Input: part model. Units: mm. Frame: model coordinates. A direction names the side the tool comes from. Round coordinates to 2 decimals unless told otherwise and drop trailing zeros. Loops run counter-clockwise (first coordinate to the right, second up) from the corner with the lowest first, then second, coordinate; pieces in that order, holes last. Notation, with made-up numbers: M -20,39 L -7,39 A29 ccw -7,72 Z; hole C -24,71.5 d5. An arc over 180 degrees is marked long. Return JSON: item names as keys, results as strings. Group by question number.
1) Contact query for flat-ended pins moving along their axis: P1, Ø2, axis at y = 7.5, z = -35.5, coming from the +X side; P2, Ø7.5, axis at x = -43, z = -15.5, coming from the +Y side; P3, Ø5, axis at x = -40.5, y = 32, coming from the -Z side; P4, Ø5, axis at x = 7.5, y = 15, coming from the +Z side. Output: stop coordinate, or through.
2) Access query for faces 5 (the face through (0, 0, -42)), 6 (the face through (0, 2, -44)), 7 (the face through (36.6, 35, -17)), 8 (the face through (-42, 36, -1.65)). Directions: +Z, -Z, +X, -X, +Y, -Y. A direction counts if a zero-diameter tool reaches every point of the face in a straight line with its end or side. Return the directions, or none.
3) Material intervals for line 1 (X direction, y = 28, z = -4); line 2 (Y direction, x = -21, z = -35.5); line 3 (X direction, y = 32.5, z = -5.5), sorted ascending. Write a range as from..to.
4) Section C-C (y = 7). Output: boundary loops of the cut face in (x, z), plus the area to 3 significant figures.
5) Mould query, pull axis Y, two halves, no side actions, for faces 1 (the face through (41, 53, 0)), 2 (the face through (-40, 49, -14)), 3 (the face through (42, 2, -14)), 4 (the face through (-41, 36, -5.65)). Classes: +Y half, -Y half, draft (parallel to the pull), parting line (faces both ways), or undercut.
6) Section B-B (y = 23.5). Output: boundary loops of the cut face in (x, z).
7) Section A-A (y = 42.5). Output: boundary loops of the cut face in (x, z).
from build123d import *

# Parameters (mm, degrees)
EXTRUDE_1_DEPTH          = 58
FILLET_1_R               = 5
SKETCH_2_W               = 14.1984483
SKETCH_2_H               = 27
CUT_EXTRUDE_1_DEPTH      = 1.65
CUT_EXTRUDE_START        = -22.111141
SKETCH_3_R               = 1.5
CUT_EXTRUDE_2_DEPTH      = 22.111141
SKETCH_5_W               = 9.9
SKETCH_5_H               = 27
CUT_EXTRUDE_3_DEPTH      = 22.65
FILLET_2_R               = 1
EXTRUDE_2_DEPTH          = 10
SKETCH_9_R               = 1
CUT_EXTRUDE_4_DEPTH      = 2
PATTERN_CIRCULAR_1_COUNT = 5


with BuildPart() as part:
    # 草图1 → 凸台-拉伸1 (new body)
    with BuildSketch(Plane(origin=(0, 0, 0), x_dir=(1, 0, 0), z_dir=(0, 1, 0))):
        with BuildLine():
            Line((-46.5, 0), (-36.6, 0))
            ThreePointArc((-36.6, 0), (0, 36.6), (36.6, 0))
            Line((36.6, 0), (46.5, 0))
            ThreePointArc((46.5, 0), (0, 46.5), (-46.5, 0))
        make_face()
    extrude(amount=EXTRUDE_1_DEPTH)

    # 圆角1
    fillet_1_edges = [part.edges().sort_by_distance(p)[0] for p in [
        (0, 0, -36.6),
    ]]
    fillet(fillet_1_edges, radius=FILLET_1_R)

    # 草图2 → 切除-拉伸1 (cut)
    with BuildSketch(Plane.XY):
        with Locations((-41.149885232, 35.5)):
            Rectangle(SKETCH_2_W, SKETCH_2_H)
    cut_extrude_1 = extrude(amount=-CUT_EXTRUDE_1_DEPTH, mode=Mode.SUBTRACT)

    # 草图3 → 切除-拉伸2 (cut)
    with BuildSketch(Plane.XY.offset(-1.65).offset(CUT_EXTRUDE_START)):
        with Locations((-41.470716586, 28.5)):
            Circle(SKETCH_3_R)
        with Locations((-41.470716586, 42.5)):
            Circle(SKETCH_3_R)
    cut_extrude_2 = extrude(amount=CUT_EXTRUDE_2_DEPTH, mode=Mode.SUBTRACT)

    # 草图5 → 切除-拉伸3 (cut)
    with BuildSketch(Plane.XY.offset(-5.65)):
        with Locations((-41.55, 35.5)):
            Rectangle(SKETCH_5_W, SKETCH_5_H)
    cut_extrude_3 = extrude(amount=-CUT_EXTRUDE_3_DEPTH, mode=Mode.SUBTRACT)

    # 镜向2: 切除-拉伸1, 切除-拉伸2, 切除-拉伸3 across plane
    add(cut_extrude_1.mirror(Plane(origin=(0, 0, 0), x_dir=(0, 0, 1), z_dir=(1, 0, 0))), mode=Mode.SUBTRACT)
    add(cut_extrude_2.mirror(Plane(origin=(0, 0, 0), x_dir=(0, 0, 1), z_dir=(1, 0, 0))), mode=Mode.SUBTRACT)
    add(cut_extrude_3.mirror(Plane(origin=(0, 0, 0), x_dir=(0, 0, 1), z_dir=(1, 0, 0))), mode=Mode.SUBTRACT)

    # 圆角2
    fillet_2_edges = [part.edges().sort_by_distance(p)[0] for p in [
        (0, 58, -46.5),
    ]]
    fillet(fillet_2_edges, radius=FILLET_2_R)

    # 草图8 → 凸台-拉伸2 (add)
    with BuildSketch(Plane.XZ):
        with BuildLine():
            Line((0, -41.6), (0, -46.5))
            ThreePointArc((0, -46.5), (-2.433621965, -46.436273366), (-4.860573542, -46.245268135))
            Line((-4.860573542, -46.245268135), (-4.348384072, -41.372110847))
            ThreePointArc((-4.348384072, -41.372110847), (-2.17717578, -41.542988646), (0, -41.6))
        make_face()
    extrude(amount=-EXTRUDE_2_DEPTH)

    # 草图9 → 切除-拉伸4 (cut)
    with BuildSketch(Plane.XZ):
        with Locations((0, -44.5)):
            Circle(SKETCH_9_R)
    cut_extrude_4 = extrude(amount=-CUT_EXTRUDE_4_DEPTH, mode=Mode.SUBTRACT)

    # 阵列(圆周)1: 切除-拉伸4 ×5 about axis
    pattern_circular_1_axis = Axis((0, 0, 0), (0, 1, 0))
    for i in range(1, PATTERN_CIRCULAR_1_COUNT):
        add(cut_extrude_4.rotate(pattern_circular_1_axis, i * 360 / PATTERN_CIRCULAR_1_COUNT), mode=Mode.SUBTRACT)


solid = part.part
Returned:
{
 "1": {"P1": "stops at x = 31.18", "P2": "stops at y = 58", "P3": "stops at z = -5.65", "P4": "stops at z = -35.21"},
 "2": {"face 5": "+Z, -Z, +X, -X, -Y", "face 6": "-Y", "face 7": "+X", "face 8": "+Z, +X, -X"},
 "3": {"line 1": "x = -46.33..-42.88, -40.06..-36.38, 36.38..40.06, 42.88..46.33", "line 2": "y = 0.01..58", "line 3": "x = -46.17..-36.18, 36.18..46.17"},
 "4": {"outline": "M -46.5,0 A46.5 ccw 46.5,0 L 36.6,0 A36.6 cw -36.6,0 Z", "area": "1,290 mm^2"},
 "5": {"face 1": "draft", "face 2": "undercut", "face 3": "-Y half", "face 4": "undercut"},
 "6": {"outline": "M -46.47,-1.65 A46.5 ccw -46.16,-5.65 L -36.6,-5.65 L -36.6,-28.3 L -36.9,-28.3 A46.5 ccw 36.9,-28.3 L 36.6,-28.3 L 36.6,-5.65 L 46.16,-5.65 A46.5 ccw 46.47,-1.65 L 36.56,-1.65 A36.6 cw -36.56,-1.65 Z"},
 "7": {"outline": "M -46.47,-1.65 A46.5 ccw -46.16,-5.65 L -42.97,-5.65 L -42.97,-1.65 Z; M -39.97,-5.65 L -36.6,-5.65 L -36.6,-28.3 L -36.9,-28.3 A46.5 ccw 36.9,-28.3 L 36.6,-28.3 L 36.6,-5.65 L 39.97,-5.65 L 39.97,-1.65 L 36.56,-1.65 A36.6 cw -36.56,-1.65 L -39.97,-1.65 Z; M 42.97,-5.65 L 46.16,-5.65 A46.5 ccw 46.47,-1.65 L 42.97,-1.65 Z"}
}
